```python
from build123d import *

# Parameters (mm, degrees)
SKETCH2_W                      = 57.15
SKETCH2_H                      = 6.35
BOSS_EXTRUDE1_DEPTH            = 63.5
SKETCH3_R                      = 14.2875
CUT_EXTRUDE1_DEPTH             = 70.922121857
CHAMFER1_SIZE                  = 6.35
M5_CLEARANCE_HOLE1_D           = 5.5
FILLET1_R                      = 0.762
CUT_EXTRUDE4_DEPTH             = 1.524
CBORE_FOR_M4_SHCS2_D           = 4.5
CBORE_FOR_M4_SHCS2_CBORE_D     = 8
CBORE_FOR_M4_SHCS2_CBORE_DEPTH = 4


with BuildPart() as part:
    # Sketch2 → Boss-Extrude1 (new body)
    with BuildSketch(Plane(origin=(0, 0, 0), x_dir=(1, 0, 0), z_dir=(0, 1, 0))):
        Rectangle(SKETCH2_W, SKETCH2_H)
    extrude(amount=-BOSS_EXTRUDE1_DEPTH)

    # Sketch3 → Cut-Extrude1 (cut, through all)
    with BuildSketch(Plane.XY.offset(3.175)):
        with Locations((0, -28.8150046)):
            Circle(SKETCH3_R)
    extrude(amount=-CUT_EXTRUDE1_DEPTH, mode=Mode.SUBTRACT)

    # Chamfer1
    chamfer1_edges = [part.edges().sort_by_distance(p)[0] for p in [
        (28.575, 0, 0),
        (-28.575, 0, 0),
    ]]
    chamfer(chamfer1_edges, length=CHAMFER1_SIZE)

    # M5 Clearance Hole1 (through all)
    with Locations(Plane.XY.offset(3.175)):
        with Locations((-19.05, -50.000003124), (19.05, -50.000003124)):
            Hole(M5_CLEARANCE_HOLE1_D / 2)

    # Fillet1
    fillet1_edges = [part.edges().sort_by_distance(p)[0] for p in [
        (28.575, -63.5, 0),
        (0, -63.5, -3.175),
        (0, 0, 3.175),
        (0, 0, -3.175),
        (22.225, 0, 0),
        (-22.225, 0, 0),
        (25.4, -3.175, 3.175),
        (-25.4, -3.175, 3.175),
        (-28.575, -6.35, 0),
        (25.4, -3.175, -3.175),
        (-25.4, -3.175, -3.175),
        (28.575, -6.35, 0),
        (-28.575, -63.5, 0),
        (-28.575, -34.925, -3.175),
        (28.575, -34.925, -3.175),
        (28.575, -34.925, 3.175),
        (-28.575, -34.925, 3.175),
        (0, -63.5, 3.175),
    ]]
    fillet(fillet1_edges, radius=FILLET1_R)

    # Sketch8 → Cut-Extrude4 (cut)
    with BuildSketch(Plane.XY.offset(3.175)):
        with BuildLine():
            Line((11.55, -63.5), (11.55, -49.5))
            ThreePointArc((11.55, -49.5), (19.05, -42), (26.55, -49.5))
            Line((26.55, -49.5), (26.55, -63.5))
            Line((26.55, -63.5), (11.55, -63.5))
        make_face()
    cut_extrude4 = extrude(amount=-CUT_EXTRUDE4_DEPTH, mode=Mode.SUBTRACT)

    # Mirror1: Cut-Extrude4 across plane
    add(cut_extrude4.mirror(Plane(origin=(0, 0, 0), x_dir=(0, 0, 1), z_dir=(1, 0, 0))), mode=Mode.SUBTRACT)

    # CBORE for M4 SHCS2 (through all)
    with Locations(Plane.XY.offset(3.175)):
        with Locations((-17.9605178, -10.8544868)):
            CounterBoreHole(CBORE_FOR_M4_SHCS2_D / 2, CBORE_FOR_M4_SHCS2_CBORE_D / 2, CBORE_FOR_M4_SHCS2_CBORE_DEPTH)


solid = part.part
```
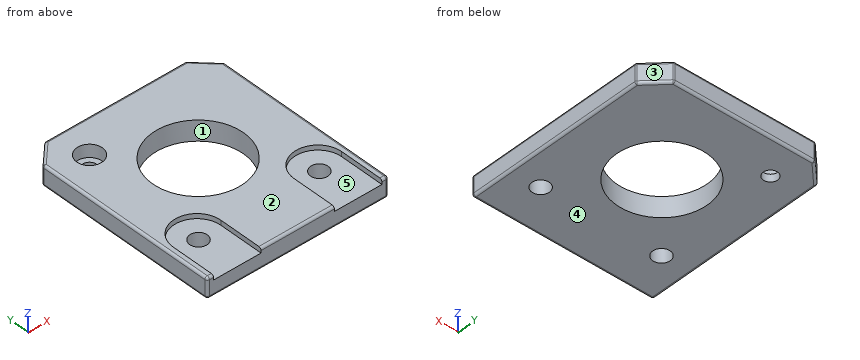
Input: part model. Units: mm. Frame: model coordinates. Face numbers are marked on the shaded views. A direction names the side the tool comes from. Coordinates: 2 decimals unless noted, no trailing zeros. Write each loop counter-clockwise with the first axis right and the second up, starting at its lowest first coordinate (ties: lowest second). Pieces come first, ordered by that corner, then holes. Notation, with made-up numbers: (27, 66) - (72, 66) arc R8 cw to (72, 70) - close; hole circle Ø3 at (51.25, 33). An arc over 180 degrees is marked (long way). Put each result on its own line as item: value. Start each with the question number.
1) Cut plane D-D (x = 19.05). Return the cut outline in (y, z) (3 decimals).
2) Mould query, pull axis Y, two halves, no side actions, for the marked faces 1, 2 and 3. Classes: pulls with the +Y half, pulls with the -Y half, needs draft (parallel to the pull), parting line crosses it, or undercut.
3) Cut plane C-C (z = 0). State how many separate pieces and enclosed holes the cut face has, plus the area to 3 significant figures.
4) Reachability of the marked faces 4 and 5 from +Z, -Z, +X, -X, +Y, -Y: full face, straight path, thin tool, end or side. Return the list, or none.
5) Cut plane B-B (y = -40). Return the cut outline in (x, z) (3 decimals), plus the area to 3 significant figures.
6) Contact query for flat-ended pins moving along their axis: pin 1 (17 mm diameter, centred on x = 0, y = -28.82, fed in from -Z); pin 2 (5 mm diameter, centred on x = -17.96, y = -10.85, fed in from +Z) (3 decimals); pin 3 (12 mm diameter, centred on x = -19, y = -57, fed in from +Z). Output: stop coordinate, or through.
7) Ray query, L1, parallel to X at y = -29, z = -1 (3 decimals); L2, parallel to Y at x = -18.5, z = -2.5; L3, parallel to X at y = -52, z = 3. Return the intervals inside material, ascending.
8) Cut plane A-A (x = 0). Return the cut outline in (y, z) (1 decimal), plus the area to 3 significant figures.
Resolved:
1. outline: (-63.5, -2.413) arc R0.762 ccw to (-62.738, -3.175) - (-52.75, -3.175) - (-52.75, 1.651) - (-63.5, 1.651) - close; (-47.25, -3.175) - (-0.762, -3.175) arc R0.762 ccw to (0, -2.413) - (0, 2.413) arc R0.762 ccw to (-0.762, 3.175) - (-42, 3.175) - (-42, 1.651) - (-47.25, 1.651) - close
2. face 1: undercut
2. face 2: needs draft
2. face 3: pulls with the +Y half
3. separate pieces: 1
3. enclosed holes: 4
3. area: 2,850 mm2
4. face 4: -Z, +X, -X, +Y, -Y
4. face 5: +Z, -Y
5. outline: (-28.575, -2.413) arc R0.762 ccw to (-27.813, -3.175) - (-8.89, -3.175) - (-8.89, 3.175) - (-27.813, 3.175) arc R0.762 ccw to (-28.575, 2.413) - close; (8.89, -3.175) - (27.813, -3.175) arc R0.762 ccw to (28.575, -2.413) - (28.575, 2.413) arc R0.762 ccw to (27.813, 3.175) - (8.89, 3.175) - close
5. area: 250 mm2
6. pin 1: passes through
6. pin 2: stops at z = -0.825
6. pin 3: stops at z = 1.65
7. L1: x = -28.575 to -14.286, 14.286 to 28.575
7. L2: y = -63.5 to -52.69, -47.31 to -13.04, -8.67 to 0
7. L3: x = -28.3 to -26.55, -11.55 to 11.55, 26.55 to 28.3
8. outline: (-63.5, -2.4) arc R0.8 ccw to (-62.7, -3.2) - (-43.1, -3.2) - (-43.1, 3.2) - (-62.7, 3.2) arc R0.8 ccw to (-63.5, 2.4) - close; (-14.5, -3.2) - (-0.8, -3.2) arc R0.8 ccw to (0, -2.4) - (0, 2.4) arc R0.8 ccw to (-0.8, 3.2) - (-14.5, 3.2) - close
8. area: 221 mm2
